Verification items for the finished model (mm, model axes). Face numbers are marked on the shaded views. A direction names the side the tool comes from. Round coordinates to 2 decimals unless told otherwise and drop trailing zeros. Write each loop counter-clockwise with the first axis right and the second up, starting at its lowest first coordinate (ties: lowest second). Pieces come first, ordered by that corner, then holes. Notation, with made-up numbers: M 64.5,71 L 89.5,71 A15 ccw 89.5,99 Z; hole C 21,66.5 d3. An arc over 180 degrees is marked long. One line per item, written item: value. Start each with the question number.
Item 1: Gauge pin test, flat ends, axial feed: pin 1 (12 mm diameter, centred on x = -2, y = -3, fed in from -Z); pin 2 (17.5 mm diameter, centred on x = 21, y = -6, fed in from +Z). Record the tip position at first contact, or that the pin passes through.
Item 2: Section check C-C, the plane y = -21.5. Record the cut outline in (x, z).
Item 3: Draft check along X on the marked faces 3, 4 and 5. Enter one of: +X half, -X half, draft (parallel to the pull), parting line (faces both ways), or undercut.
Item 4: Thickness scan on probe 1 along X at (y, z) = (-14, 12); probe 2 along Y at (x, z) = (38.5, 3); probe 3 along Z at (x, y) = (42.5, 11). Record the ranges inside material, lowest first. Write a range as from..to.
Item 5: Section check B-B, the plane z = 25.5. Record the cut outline in (x, y), then the cut area to 3 significant figures.
Item 6: Section check D-D, the plane z = 38.5. Record the cut outline in (x, y).
Item 7: Section check A-A, the plane x = 53. Record the cut outline in (y, z), then the cut area to 3 significant figures.
Item 8: Tool access check on the marked faces 1 and 2. Record the directions out of +Z, -Z, +X, -X, +Y, -Y that give a thin tool (end or side, any length) a straight path to the whole face; none if there is none.
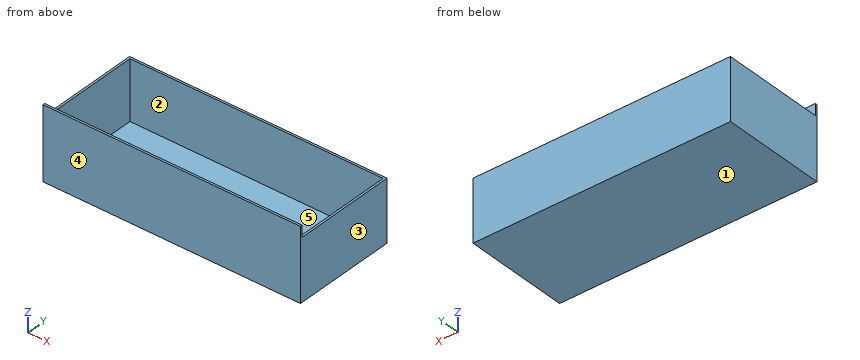
from build123d import *

# Parameters (mm, degrees)
F0_W     = 147
F0_H     = 60
F1_DEPTH = 35
F2_W     = 147
F2_H     = 1.6
F3_DEPTH = 6.5
F4_T     = -1.2
F5_DEPTH = 0.4


# Not quite as in the source:
# - a shell that OpenCascade refuses in one call is made with other operations: the cavity is built on its own and cut out


with BuildPart() as f1:
    # F0 (on Top) → F1 (new body)
    with BuildSketch(Plane.XY):
        with Locations((2.3024454713, -14.3951082311)):
            Rectangle(F0_W, F0_H)
    extrude(amount=F1_DEPTH)

    # F2 (on face) → F3 (join)
    with BuildSketch(Plane.XY.offset(35)):
        with Locations((2.3024454713, -43.5951082311)):
            Rectangle(F2_W, F2_H)
    extrude(amount=F3_DEPTH)

    # F4: a shell. OpenCascade refuses it in one call, so the cavity is built on its own and cut out:
    # the body offset inwards by the wall thickness, plus a prism from it out through each open face.
    f4_core = offset(f1.part, amount=F4_T, kind=Kind.INTERSECTION, mode=Mode.PRIVATE)
    f4_exits = [f4_core.faces().sort_by_distance(p)[0] for p in [
        (2.302445, -14.395108, 33.8),
    ]]
    add(f4_core, mode=Mode.SUBTRACT)
    extrude(f4_exits, amount=-F4_T, mode=Mode.SUBTRACT)

    # F5 (cut): a face of the model
    f5_faces = [f1.faces().sort_by_distance(p)[0] for p in [
        (2.3024454713, -42.7951082311, 38.25),
    ]]
    extrude(f5_faces, amount=-F5_DEPTH, mode=Mode.SUBTRACT)


solid = f1.part
Response values:
1. pin 1: stops at z = 0
1. pin 2: stops at z = 1.2
2. outline: M -71.2,0 L 75.8,0 L 75.8,35 L 74.6,35 L 74.6,1.2 L -70,1.2 L -70,35 L -71.2,35 Z
3. face 3: +X half
3. face 4: draft
3. face 5: undercut
4. probe 1: x = -71.2..-70, 74.6..75.8
4. probe 2: y = -44.4..-43.2, 14.4..15.6
4. probe 3: z = 0..1.2
5. outline: M -71.2,-44.4 L 75.8,-44.4 L 75.8,15.6 L -71.2,15.6 Z; hole M -70,-43.2 L 74.6,-43.2 L 74.6,14.4 L -70,14.4 Z
5. area: 491 mm2
6. outline: M -71.2,-44.4 L 75.8,-44.4 L 75.8,-43.2 L -71.2,-43.2 Z
7. outline: M -44.4,0 L 15.6,0 L 15.6,35 L 14.4,35 L 14.4,1.2 L -43.2,1.2 L -43.2,41.5 L -44.4,41.5 Z
7. area: 161 mm2
8. face 1: -Z, +X, -X, +Y, -Y
8. face 2: +Z
